Autodesk Inventor part; units mm, degrees
ref_plane "YZ Plane" through (0, 0, 0) normal (1, 0, 0) x (0, 1, 0)
ref_plane "XZ Plane" through (0, 0, 0) normal (0, 1, 0) x (-1, 0, 0)
ref_plane "XY Plane" through (0, 0, 0) normal (0, 0, 1) x (1, 0, 0)
sketch "Sketch1" plane through (0, 0, 0) normal (1, 0, 0) x (0, 1, 0)
  line L0 (0, 0) -> (25.4, 0)
  line L1 (25.4, 0) -> (25.4, -50.8)
  line L2 (25.4, -50.8) -> (0, -50.8)
  line L3 (0, -50.8) -> (0, 0)
  line L4 (22.225, -47.625) -> (22.225, -3.175)
  line L5 (22.225, -3.175) -> (3.175, -3.175)
  line L6 (3.175, -3.175) -> (3.175, -47.625)
  line L7 (3.175, -47.625) -> (22.225, -47.625)
  dimension "d0" = 25.4
  dimension "d1" = 50.8
  dimension "d2" = 3.175
extrude "Extrusion1" add sketch "Sketch1" along normal blind 130.175
sketch "Sketch2" plane through (0, 0, -50.8) normal (0, -1, 0) x (1, 0, 0)
  circle A0 centre (114.3, 22.225) radius 3.175
  circle A1 centre (98.425, 38.1) radius 3.175
  line L0 (130.175, 50.8) -> (130.175, 0)
  line L1 (0, 50.8) -> (130.175, 50.8)
  circle A2 centre (9.525, 12.7) radius 3.175
  circle A3 centre (9.525, 38.1) radius 3.175
  circle A4 centre (28.575, 12.7) radius 3.175
  circle A5 centre (28.575, 38.1) radius 3.175
  line L2 (0, 0) -> (0, 50.8)
  line L3 (0, 0) -> (130.175, 0)
  dimension "d5" = 6.35
  dimension "d6" = 6.35
  dimension "d7" = 31.75
  dimension "d8" = 15.875
  dimension "d9" = 28.575
  dimension "d10" = 12.7
  dimension "d13" = 6.35
  dimension "d14" = 6.35
  dimension "d15" = 6.35
  dimension "d16" = 6.35
  dimension "d17" = 12.7
  dimension "d18" = 12.7
  dimension "d19" = 9.525
  dimension "d20" = 9.525
  dimension "d21" = 12.7
  dimension "d22" = 12.7
  dimension "d23" = 25.4
  dimension "d24" = 28.575
extrude "Extrusion2" cut sketch "Sketch2" against normal blind 25.4 contours A0 | A1 | A2 | A3 | A4 | A5
properties part number "15102898-16-P-0801" material "Aluminum 6061"
Can you work these out from the model? Positions are in its coordinate system, mm. A direction names the side the tool comes from. Round coordinates to 2 decimals unless told otherwise and drop trailing zeros. Loops run counter-clockwise (first coordinate to the right, second up) from the corner with the lowest first, then second, coordinate; pieces in that order, holes last. Notation, with made-up numbers: (50.5, -15.5) - (58.5, -15.5) arc R29 cw to (58.5, 7.5) - close; hole circle Ø10 at (-0.5, -38.5). An arc over 180 degrees is marked (long way). Answer in a Markdown table with one row per item. Add a question column.
Q1. We'd pull the mould along Y, two halves only. Please class faces 1 (the flat face through (64, 25.4, -25)), 2 (the flat face through (64, 0, -26)), 3 (the flat face through (64, 22.225, -26)), 4 (the cylindrical face through (12.458, 23.79, -13.916)): pulls with the +Y half, pulls with the -Y half, needs draft (parallel to the pull), parting line crosses it, or undercut.
Q2. I need wall thicknesses on L1, parallel to Y at x = 108, z = -42.5 (3 decimals); L2, parallel to Z at x = 16.5, y = 22 (3 decimals); L3, parallel to Z at x = 114.3, y = 1.65. Which ranges of each line are inside material? Lowest first, please.
Q3. For pin 1 Ø7.5 at (x, z) = (28.575, -38.1) entering from +Y, with a flat end and sliding along its axis, tell me the tip position at first contact or that it passes through.
Q4. Which directions (+Z, -Z, +X, -X, +Y, -Y) give clear straight access to the entire face, cutting with the end or side of a thin tool? Please do faces 5 (the flat face through (64, 13, 0)), 6 (the flat face through (64, 13, -3.175)).
Q5. I want a section at B-B on z = -12.7. Count the separate pieces of the cut face and the enclosed holes in it, and give its area (3 significant figures).
Q6. I want a section at A-A on y = 6. List the corners of the cut face in (x, z) for me (3 decimals).
Q7. I want a section at C-C on x = 114.3. List the corners of the cut face in (y, z) for me (3 decimals).
Q8. I want a section at D-D on z = -38.1. List the corners of the cut face in (x, y) for me (3 decimals).
A:
| question | item | result |
|---|---|---|
| 1 | face 1 | pulls with the +Y half |
| 1 | face 2 | pulls with the -Y half |
| 1 | face 3 | undercut |
| 1 | face 4 | needs draft |
| 2 | L1 | 0 to 3.175, 22.225 to 25.4 |
| 2 | L2 | -50.8 to -47.625, -3.175 to 0 |
| 2 | L3 | -50.8 to -31.75, -25.4 to 0 |
| 3 | pin 1 | y = 25.4 |
| 4 | face 5 | +Z, +X, -X, +Y, -Y |
| 4 | face 6 | +X, -X |
| 5 | separate pieces | 8 |
| 5 | enclosed holes | 0 |
| 5 | area | 706 mm^2 |
| 6 | outline | (0, -50.8) - (130.175, -50.8) - (130.175, -47.625) - (0, -47.625) - close; (0, -3.175) - (130.175, -3.175) - (130.175, 0) - (0, 0) - close |
| 7 | outline | (0, -50.8) - (25.4, -50.8) - (25.4, -31.75) - (22.225, -31.75) - (22.225, -47.625) - (3.175, -47.625) - (3.175, -31.75) - (0, -31.75) - close; (0, -25.4) - (3.175, -25.4) - (3.175, -3.175) - (22.225, -3.175) - (22.225, -25.4) - (25.4, -25.4) - (25.4, 0) - (0, 0) - close |
| 8 | outline | (0, 0) - (6.35, 0) - (6.35, 3.175) - (0, 3.175) - close; (0, 22.225) - (6.35, 22.225) - (6.35, 25.4) - (0, 25.4) - close; (12.7, 0) - (25.4, 0) - (25.4, 3.175) - (12.7, 3.175) - close; (12.7, 22.225) - (25.4, 22.225) - (25.4, 25.4) - (12.7, 25.4) - close; (31.75, 0) - (130.175, 0) - (130.175, 3.175) - (31.75, 3.175) - close; (31.75, 22.225) - (130.175, 22.225) - (130.175, 25.4) - (31.75, 25.4) - close |
